from build123d import *


with BuildPart() as part:
    # 草图1 → 旋转1 (revolve)
    with BuildSketch(Plane(origin=(0, 0, 0), x_dir=(1, 0, 0), z_dir=(0, 1, 0)), mode=Mode.PRIVATE) as revolve_1_sk:
        Polygon((0, 0), (0, 7.5), (9, 7.5), (9, 6.9), (10, 6.9), (10, 7.5), (18, 7.5), (18, 8.5), (159, 8.5), (159, 7.85), (160, 7.85), (160, 8.5), (190, 8.5), (190, 10), (286.5, 10), (286.5, 8.5), (294.5, 8.5), (294.5, 0), align=None)
    revolve(revolve_1_sk.sketch.rotate(Axis((-79.560771626, 0, 0), (1, 0, 0)), 180), axis=Axis((-79.560771626, 0, 0), (1, 0, 0)))


solid = part.part
Work out the finished part from the listing and answer in its coordinate system (mm). A direction names the side the tool comes from. Round coordinates to 2 decimals unless told otherwise and drop trailing zeros. Order: outer loops, then holes, each group sorted by start corner. A loop starts at its lowest first (then second) coordinate and runs counter-clockwise, first axis right, second up. Notation, with made-up numbers: M -5.75,-19 L 27.25,-19 A21 ccw 27.25,13 Z; hole C -15,76.25 d3. An arc over 180 degrees is marked long. Put each result on its own line as item: value. Start each with the question number.
Q1. For a pull along X with two mould halves and no side action, classify faces 1 (the flat face through (294.5, 0, 0)), 2 (the cylindrical face through (290.556, -8.428, -1.107)), 3 (the cylindrical face through (9.51, -4.66, -5.09)) as pulls with the +X half, pulls with the -X half, needs draft (parallel to the pull), parting line crosses it, or undercut.
Q2. Section D-D, the plane x = 62.5 is taken. Write down the section's boundary in (y, z).
Q3. Straight lines are drawn through the part: L1, parallel to Z at x = 101, y = 1; L2, parallel to X at y = 4, z = 7; L3, parallel to Y at x = 252.5, z = -5.25. For each, find the intervals that lie inside material, in ascending order. Write a range as [from, to].
Q4. Section C-C, the plane x = 259 is taken. Write down the section's boundary in (y, z).
Q5. A tool of negligible diameter and unlimited length cuts with its end or side. For faces 4 (the flat face through (286.5, 7.4, -4.5)), 5 (the flat face through (9, 7, 2)), 6 (the cylindrical face through (239, 0, -10)), 7 (the cylindrical face through (175.21, -8.428, -1.107)), from which of +Z, -Z, +X, -X, +Y, -Y can it reach the whole face along a straight path? Write none if from no direction.
Q6. Flat-ended cylindrical pins translate along their axes: pin 1 (6 mm diameter, centred on x = 79, y = 0.5, fed in from -Z); pin 2 (3 mm diameter, centred on y = -7.5, z = -3.5, fed in from -X); pin 3 (4 mm diameter, centred on x = 140.5, z = -6.5, fed in from +Y); pin 4 (1 mm diameter, centred on x = 146.5, z = 6, fed in from +Y). Find the tip coordinate at first contact, or state that the pin passes through.
Findings below:
1. face 1: pulls with the +X half
1. face 2: needs draft
1. face 3: undercut
2. outline: C 0,0 d17
3. L1: z = [-8.44, 8.44]
3. L2: x = [18, 159], [160, 294.5]
3. L3: y = [-8.51, 8.51]
4. outline: C 0,0 d20
5. face 4: +X
5. face 5: none
5. face 6: +X, -X
5. face 7: -X
6. pin 1: stops at z = -8.5
6. pin 2: stops at x = 0
6. pin 3: stops at y = 7.21
6. pin 4: stops at y = 6.48
